Model file for the job. Use its own axes, mm. Face numbers are marked on the shaded views. A direction names the side the tool comes from. Round coordinates to 2 decimals unless told otherwise and drop trailing zeros. Loops run counter-clockwise (first coordinate to the right, second up) from the corner with the lowest first, then second, coordinate; pieces in that order, holes last. Notation, with made-up numbers: M 7,6 L 56,6 A10 ccw 56,18 Z; hole C 33,43.5 d1. An arc over 180 degrees is marked long. Use a Markdown table: item, result. Add a question column.
Q1. Tool access for the marked faces 1, 2, 3, 4 and 5: list every direction of +Z, -Z, +X, -X, +Y, -Y with a clear straight run to the whole face (end or side of a thin tool).
Q2. Pin check, flat tips, straight feed: pin 1 (5 mm diameter, centred on x = 20.2, y = 20.2, fed in from -Z); pin 2 (3 mm diameter, centred on x = -17.5, z = 29, fed in from -Y); pin 3 (10 mm diameter, centred on x = 4.5, z = -1.5, fed in from +Y); pin 4 (4 mm diameter, centred on x = -17, y = 33.5, fed in from +Z). Stop position of each tip, or through.
Q3. Mould opens along X. For the marked faces 6, 7 and 8 say: +X half, -X half, draft (parallel to the pull), parting line (faces both ways), or undercut.
Q4. Probe line 1 (Z direction, x = -9.5, y = 6); line 2 (X direction, y = -20, z = -2); line 3 (X direction, y = -3.5, z = -7.5). List the from-to ranges inside material, lowest first. Write a range as from..to.
Q5. Cut at B-B (z = 8.5). Give the cut face in (x, y).
Q6. Cut at C-C (y = 25.5). Give the cut face in (x, z).
Q7. Cut at A-A (y = 12). Give the cut face in (x, z).
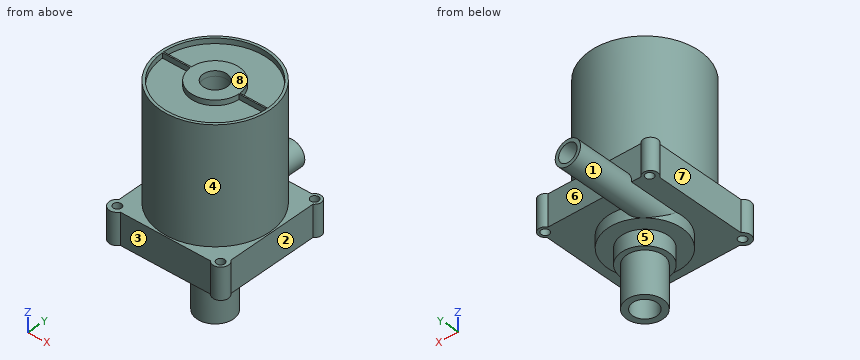
from build123d import *

# Parameters (mm, degrees)
SKETCH2_R                 = 21
BOSS_EXTRUDE4_DEPTH       = 44
SKETCH6_R                 = 2.52099285
SKETCH6_R_2               = 2.774223213
SKETCH6_R_3               = 2.958692603
SKETCH6_R_4               = 3.108326591
SKETCH6_W                 = 43
SKETCH6_H                 = 43
BOSS_EXTRUDE8_DEPTH       = 12
SKETCH7_R                 = 1.557999949
CUT_EXTRUDE1_DEPTH        = 12
SKETCH9_R                 = 14.25
BOSS_EXTRUDE10_DEPTH      = 4.5
SKETCH10_R                = 4.856031572
BOSS_EXTRUDE12_DEPTH      = 22
BOSS_EXTRUDE12_DEPTH_BACK = 22
SKETCH11_R                = 9
BOSS_EXTRUDE13_DEPTH      = 6
SKETCH12_R                = 7
BOSS_EXTRUDE14_DEPTH      = 16
SKETCH13_R                = 4.670506922
CUT_EXTRUDE3_DEPTH        = 120
SKETCH15_R                = 3.527063208
CUT_EXTRUDE5_DEPTH        = 40
SKETCH16_R                = 20
CUT_EXTRUDE6_DEPTH        = 2
SKETCH17_W                = 40.997064224
SKETCH17_H                = 0.490637438
BOSS_EXTRUDE15_DEPTH      = 2
SKETCH18_R                = 9.319375459
BOSS_EXTRUDE16_DEPTH      = 2
SKETCH19_R                = 4.582310756
CUT_EXTRUDE7_DEPTH        = 2


with BuildPart() as part:
    # Sketch2 → Boss-Extrude4 (new body)
    with BuildSketch(Plane.XY):
        Circle(SKETCH2_R)
    extrude(amount=BOSS_EXTRUDE4_DEPTH)

    # Sketch6 → Boss-Extrude8 (add)
    with BuildSketch(Plane(origin=(0, 0, 0), x_dir=(-1, 0, 0), z_dir=(0, 0, -1))):
        with Locations((-20.202035706, 20.202035706)):
            Circle(SKETCH6_R)
        with Locations((19.846366063, 19.846366063)):
            Circle(SKETCH6_R_2)
        with Locations((-19.561830349, -19.561830349)):
            Circle(SKETCH6_R_3)
        with Locations((19.846366063, -19.846366063)):
            Circle(SKETCH6_R_4)
        Rectangle(SKETCH6_W, SKETCH6_H)
    extrude(amount=BOSS_EXTRUDE8_DEPTH)

    # Sketch7 → Cut-Extrude1 (cut)
    with BuildSketch(Plane(origin=(0, 0, -12), x_dir=(-1, 0, 0), z_dir=(0, 0, -1))):
        with Locations((-20.202035706, 20.202035706)):
            Circle(SKETCH7_R)
        with Locations((19.832590029, 20.202035706)):
            Circle(SKETCH7_R)
        with Locations((19.846366063, -19.846366063)):
            Circle(SKETCH7_R)
        with Locations((-19.76209834, -19.846366063)):
            Circle(SKETCH7_R)
    extrude(amount=-CUT_EXTRUDE1_DEPTH, mode=Mode.SUBTRACT)

    # Sketch9 → Boss-Extrude10 (add)
    with BuildSketch(Plane(origin=(0, 0, -12), x_dir=(-1, 0, 0), z_dir=(0, 0, -1))):
        Circle(SKETCH9_R)
    extrude(amount=BOSS_EXTRUDE10_DEPTH)

    # Sketch10 → Boss-Extrude12 (add, two sides)
    with BuildSketch(Plane(origin=(0, 21.5, 0), x_dir=(1, 0, 0), z_dir=(0, 1, 0))) as boss_extrude12_sk:
        with Locations((-9.192655729, 11.573586892)):
            Circle(SKETCH10_R)
    extrude(amount=BOSS_EXTRUDE12_DEPTH)
    extrude(boss_extrude12_sk.sketch, amount=-BOSS_EXTRUDE12_DEPTH_BACK)

    # Sketch11 → Boss-Extrude13 (add)
    with BuildSketch(Plane(origin=(0, 0, -16.5), x_dir=(-1, 0, 0), z_dir=(0, 0, -1))):
        Circle(SKETCH11_R)
    extrude(amount=BOSS_EXTRUDE13_DEPTH)

    # Sketch12 → Boss-Extrude14 (add)
    with BuildSketch(Plane(origin=(0, 0, -22.5), x_dir=(-1, 0, 0), z_dir=(0, 0, -1))):
        Circle(SKETCH12_R)
    extrude(amount=BOSS_EXTRUDE14_DEPTH)

    # Sketch13 → Cut-Extrude3 (cut)
    with BuildSketch(Plane(origin=(0, 0, -38.5), x_dir=(-1, 0, 0), z_dir=(0, 0, -1))):
        Circle(SKETCH13_R)
    extrude(amount=-CUT_EXTRUDE3_DEPTH, mode=Mode.SUBTRACT)

    # Sketch15 → Cut-Extrude5 (cut)
    with BuildSketch(Plane(origin=(0, 43.5, 0), x_dir=(1, 0, 0), z_dir=(0, 1, 0))):
        with Locations((-9.192655729, 11.573586892)):
            Circle(SKETCH15_R)
    extrude(amount=-CUT_EXTRUDE5_DEPTH, mode=Mode.SUBTRACT)

    # Sketch16 → Cut-Extrude6 (cut)
    with BuildSketch(Plane.XY.offset(44)):
        Circle(SKETCH16_R)
    extrude(amount=-CUT_EXTRUDE6_DEPTH, mode=Mode.SUBTRACT)

    # Sketch17 → Boss-Extrude15 (add)
    with BuildSketch(Plane.XY.offset(42)):
        Rectangle(SKETCH17_W, SKETCH17_H)
    extrude(amount=BOSS_EXTRUDE15_DEPTH)

    # Sketch18 → Boss-Extrude16 (add)
    with BuildSketch(Plane.XY.offset(42)):
        Circle(SKETCH18_R)
    extrude(amount=BOSS_EXTRUDE16_DEPTH)

    # Sketch19 → Cut-Extrude7 (cut)
    with BuildSketch(Plane.XY.offset(44)):
        Circle(SKETCH19_R)
    extrude(amount=-CUT_EXTRUDE7_DEPTH, mode=Mode.SUBTRACT)


solid = part.part
Checked values:
| question | item | result |
|---|---|---|
| 1 | face 1 | +Y |
| 1 | face 2 | +Z, -Z, +X |
| 1 | face 3 | +Z, -Z, -Y |
| 1 | face 4 | +Z |
| 1 | face 5 | -Z |
| 2 | pin 1 | stops at z = -12 |
| 2 | pin 2 | stops at y = -13.6 |
| 2 | pin 3 | stops at y = 21.5 |
| 2 | pin 4 | passes through |
| 3 | face 6 | undercut |
| 3 | face 7 | -X half |
| 3 | face 8 | draft |
| 4 | line 1 | z = -16.5..-15.09, -8.06..42 |
| 4 | line 2 | x = -22.95..-21.4, -18.3..18.21, 21.31..22.49 |
| 4 | line 3 | x = -21.5..-3.09, 3.09..21.5 |
| 5 | outline | C 0,0 d42; hole C 0,0 d9.34 |
| 6 | outline | C -9.19,-11.57 d9.71; hole C -9.19,-11.57 d7.05 |
| 7 | outline | M -21.5,-12 L -14.03,-12 A4.86 ccw -7.69,-16.19 L -7.69,-16.5 L 7.69,-16.5 L 7.69,-12 L 21.5,-12 L 21.5,0 L 17.23,0 L 17.23,44 L 16,44 L 16,42 L -16,42 L -16,44 L -17.23,44 L -17.23,0 L -21.5,0 Z; hole C -9.19,-11.57 d7.05 |
